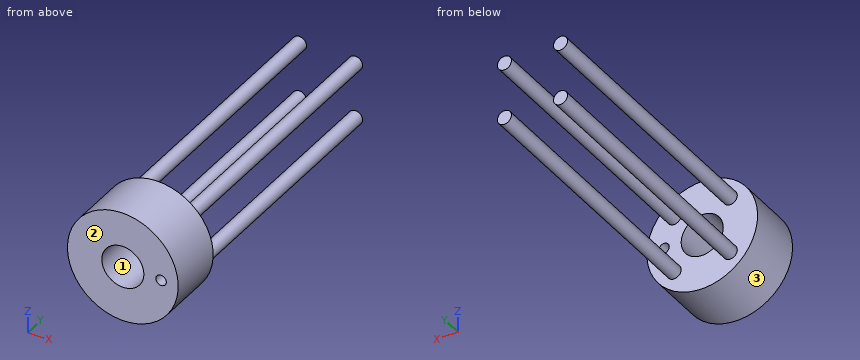
Autodesk Inventor part; units mm, degrees
ref_plane "YZ Plane" through (0, 0, 0) normal (1, 0, 0) x (0, 1, 0)
ref_plane "XZ Plane" through (0, 0, 0) normal (0, 1, 0) x (-1, 0, 0)
ref_plane "XY Plane" through (0, 0, 0) normal (0, 0, 1) x (1, 0, 0)
sketch "Sketch1" plane through (0, 0, 0) normal (0, 1, 0) x (-1, 0, 0)
  circle A0 centre (0, 0) radius 50.165
  circle A1 centre (0, 0) radius 19.05
  line L0 (0, 50.165) -> (0, -50.165)
  line L1 (50.165, 0) -> (-50.165, 0)
  line L2 (0, 0) -> (-31.75, 0)
  line L3 (0, 0) -> (-25.4, 0)
  line L4 (0, 25.4) -> (0, 0)
  circle A2 centre (-25.4, 25.4) radius 6.35
  circle A3 centre (25.4, 25.4) radius 6.35
  circle A4 centre (-25.4, -25.4) radius 6.35
  circle A5 centre (25.4, -25.4) radius 6.35
  line L5 (-19.05, 0) -> (-50.165, 0)
  circle A6 centre (-34.6075, 0) radius 4.7625
  dimension "d1" = 38.1
  dimension "d0" = 100.33
  dimension "d6" = 31.75
  dimension "d10" = 12.7
  dimension "d13" = 9.525
extrude "Extrusion1" add sketch "Sketch1" along normal blind 50.8 contours L1 A1 L0 A0 | A0 L0 A1 L1 | L0 A1 L1 A6 A0 | A0 L1 A6 A1 L0 | L1 L0 A1 | A1 L0 L1 | A1 L1 L0 | L0 L1 A1 | A6 L1 | L1 A6 | A2 | A3 | A4 | A5
extrude "Extrusion2" cut sketch "Sketch1" along normal blind 285.242 contours L1 L0 A1 | A1 L0 L1 | A1 L1 L0 | L0 L1 A1
extrude "Extrusion3" add sketch "Sketch1" along normal blind 297.561 contours A2 | A3 | A4 | A5
extrude "Extrusion4" cut sketch "Sketch1" along normal blind 79.375 contours A6 L1 | L1 A6
properties part number "Chamber Top"
Read the model definition and answer for the solid it produces. Units are mm, in the model's axes. Face numbers are marked on the shaded views. Give positions to 0.01 mm unless a question says otherwise; leave off trailing zeros. Loops run counter-clockwise (first coordinate to the right, second up) from the corner with the lowest first, then second, coordinate; pieces in that order, holes last. Notation, with made-up numbers: (-25.75, 28.5) -> (-7.75, 28.5) arc R34 ccw to (-7.75, 60.5) -> close; hole circle Ø3 at (-32, 89.25). An arc over 180 degrees is marked (long way). Use a Markdown table: item, result.
Q1. Find the intervals of material crossed by line 1 along X through (y, z) = (22, 0) (3 decimals); line 2 along X through (y, z) = (180, 25.5); line 3 along Y through (x, z) = (18.5, 33), in increasing order.
Solved:
| item | result |
|---|---|
| line 1 | x = -50.165 to -19.05, 19.05 to 29.845, 39.37 to 50.165 |
| line 2 | x = -31.75 to -19.05, 19.05 to 31.75 |
| line 3 | y = 0 to 50.8 |
Q2. Section B-B, the plane y = 217 is taken. Determine the outline of the cut face in (x, z).
Solved:
| item | result |
|---|---|
| outline | circle Ø12.7 at (-25.4, -25.4); circle Ø12.7 at (-25.4, 25.4); circle Ø12.7 at (25.4, -25.4); circle Ø12.7 at (25.4, 25.4) |
Q3. Determine the mould class of the marked faces 1, 2 and 3 for opening direction Z: pulls with the +Z half, pulls with the -Z half, needs draft (parallel to the pull), parting line crosses it, or undercut.
Solved:
| item | result |
|---|---|
| face 1 | undercut |
| face 2 | needs draft |
| face 3 | parting line crosses it |
Q4. Section A-A, the plane x = 0 is taken. Determine the outline of the cut face in (y, z) (3 decimals), then the cut area to 3 significant figures.
Solved:
| item | result |
|---|---|
| outline | (0, -50.165) -> (50.8, -50.165) -> (50.8, -19.05) -> (0, -19.05) -> close; (0, 19.05) -> (50.8, 19.05) -> (50.8, 50.165) -> (0, 50.165) -> close |
| area | 3,160 mm^2 |
Q5. Section C-C, the plane y = 34.5 is taken. Count the separate pieces of the cut face and the enclosed holes in it, then the cut area to 3 significant figures.
Solved:
| item | result |
|---|---|
| separate pieces | 1 |
| enclosed holes | 2 |
| area | 6,690 mm^2 |
Q6. Section D-D, the plane z = -25.4 is taken. Determine the outline of the cut face in (x, y).
Solved:
| item | result |
|---|---|
| outline | (-43.26, 0) -> (43.26, 0) -> (43.26, 50.8) -> (31.75, 50.8) -> (31.75, 297.56) -> (19.05, 297.56) -> (19.05, 50.8) -> (-19.05, 50.8) -> (-19.05, 297.56) -> (-31.75, 297.56) -> (-31.75, 50.8) -> (-43.26, 50.8) -> close |
Q7. Each of these flat-tipped pins is pushed along its axis until it touches: pin 1 (12 mm diameter, centred on x = 16.5, z = -34.5, fed in from -Y); pin 2 (1.5 mm diameter, centred on x = -19.5, y = 239.5, fed in from -Z); pin 3 (12 mm diameter, centred on y = 96.5, z = -9.5, fed in from -X); pin 4 (2 mm diameter, centred on x = -21.5, z = 4.5, fed in from +Y). Where does it stop, or does it pass through?
Solved:
| item | result |
|---|---|
| pin 1 | stops at y = 0 |
| pin 2 | stops at z = -29.11 |
| pin 3 | passes through |
| pin 4 | stops at y = 50.8 |
